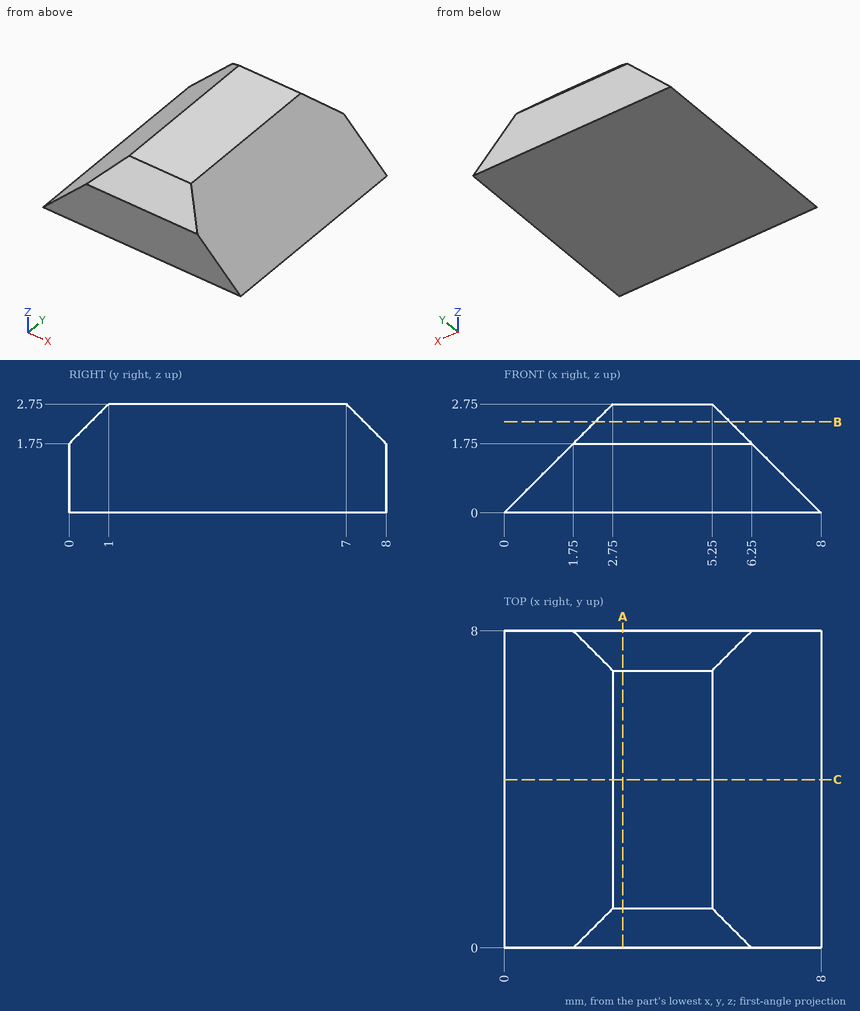
The drawing under review shows one solid part. Ordinate dimensions are in mm from its lowest x, y, z. Round coordinates to 2 decimals unless told otherwise and drop trailing zeros. Order: outer loops, then holes, each group sorted by start corner. A loop starts at its lowest first (then second) coordinate and runs counter-clockwise, first axis right, second up. Notation, with made-up numbers: (19.5, -16.5) - (67.5, -16.5) arc R35 ccw to (67.5, 19.5) - close; hole circle Ø9 at (48, 10.25). An arc over 180 degrees is marked (long way). Return JSON: item names as keys, results as strings.
Q1. Consider section A-A on x = 3. Write out the cut boundary in (y, z), plus the area to 3 significant figures.
Computed values:
{"outline": "(0, 0) - (8, 0) - (8, 1.75) - (7, 2.75) - (1, 2.75) - (0, 1.75) - close", "area": "21.0 mm2"}
Q2. Consider section C-C on y = 4.25. Write out the cut boundary in (x, z).
Computed values:
{"outline": "(0, 0) - (8, 0) - (5.25, 2.75) - (2.75, 2.75) - close"}
Q3. Consider section B-B on z = 2.3. Write out the cut boundary in (x, y).
Computed values:
{"outline": "(2.3, 0.55) - (5.7, 0.55) - (5.7, 7.45) - (2.3, 7.45) - close"}
Q4. Wall thickness on L1, parallel to Z at x = 1, y = 2; L2, parallel to X at y = 6.5, z = 1; L3, parallel to Z at x = 1.75, y = 1.25: over which ranges is each line inside the solid? List them lowest first. Write a range as [from, to].
Computed values:
{"L1": "z = [0, 1]", "L2": "x = [1, 7]", "L3": "z = [0, 1.75]"}
Q5. For pin 1 Ø1.5 at (y, z) = (5.5, 2.5) entering from +X, flat-tipped, find the tip position at first contact; note if it passes through.
Computed values:
{"pin 1": "stops at x = 6.25"}
